Autodesk Inventor part; units mm, degrees
ref_plane "YZ Plane" through (0, 0, 0) normal (1, 0, 0) x (0, 1, 0)
ref_plane "XZ Plane" through (0, 0, 0) normal (0, 1, 0) x (-1, 0, 0)
ref_plane "XY Plane" through (0, 0, 0) normal (0, 0, 1) x (1, 0, 0)
sketch "Sketch2" plane through (0, 0, 0) normal (0, 1, 0) x (-1, 0, 0)
  line L0 (-26, 25.5) -> (26, 25.5)
  line L1 (26, 25.5) -> (26, -25.5)
  line L2 (26, -25.5) -> (-26, -25.5)
  line L3 (-26, -25.5) -> (-26, 25.5)
  line L4 (-26, 25.5) -> (26, -25.5) construction
  line L5 (26, 25.5) -> (-26, -25.5) construction
  circle A0 centre (24, 23.5) radius 1
  circle A1 centre (24, -23.5) radius 1
  circle A2 centre (-24, 23.5) radius 1
  circle A3 centre (-24, -23.5) radius 1
  line L6 (10, 6) -> (-10, 6)
  line L7 (-10, -6) -> (10, -6)
  line L8 (10, 6) -> (-10, -6) construction
  line L9 (-10, 6) -> (10, -6) construction
  line L10 (10, 6) -> (10, -6)
  line L11 (-10, 6) -> (-10, -6)
  point P0 (0, 0)
  dimension "d2" = 52
  dimension "d3" = 51
  dimension "d4" = 2
  dimension "d5" = 2
  dimension "d6" = 2
  dimension "d9" = 47
  dimension "d12" = 48
  dimension "d17" = 20
  dimension "d18" = 12
extrude "Extrusion2" add sketch "Sketch2" along normal blind 1.6
equation "\"d5\" = d4"
equation "\"d6\" = d4"
properties part number "rapoukMotherboardConnectorv0"
The listing builds one solid part. Answer for the finished solid, in the listing's coordinates (mm). A direction names the side the tool comes from. Give positions to 0.01 mm unless a question says otherwise; leave off trailing zeros. Loops run counter-clockwise (first coordinate to the right, second up) from the corner with the lowest first, then second, coordinate; pieces in that order, holes last. Notation, with made-up numbers: (42.25, 18.25) - (78.25, 18.25) arc R18 cw to (78.25, 38.25) - close; hole circle Ø5 at (45, 49.25). An arc over 180 degrees is marked (long way). Answer as CSV lines item,"result". Start each with the question number.
Item 1: A cutting plane is placed at D-D on x = 3.5. Determine the outline of the cut face in (y, z).
Item 2: This flat-tipped pin is pushed along its axis until it touches: pin 1 (1.8 mm diameter, centred on x = -24, z = 23.5, fed in from +Y). Where does it stop, or does it pass through?
Item 3: Find the intervals of material crossed by line 1 (Z direction, x = 24, y = 1.05); line 2 (Z direction, x = 6.5, y = 1), in increasing order. Write a range as from..to.
Item 4: A cutting plane is placed at B-B on z = 2. Determine the outline of the cut face in (x, y).
Item 5: A cutting plane is placed at C-C on y = 0.35. Determine the outline of the cut face in (x, z), then the cut area to 3 significant figures.
Item 6: For faces 1 (the face through (10, 1, 0)), 2 (the face through (-26, 1, 0)), determine the directions among +Z, -Z, +X, -X, +Y, -Y from which every point of the face is accessible in a straight line to the end or side of a thin tool.
Item 7: The mould has two halves that part along Z. Classify faces 3 (the face through (0, 1, -25.5)), 4 (the face through (-11, 1.6, 0)), 5 (the face through (0, 1, -6)): +Z half, -Z half, draft (parallel to the pull), parting line (faces both ways), or undercut.
Item 8: A cutting plane is placed at A-A on x = 24. Determine the outline of the cut face in (y, z).
Found:
1,outline,"(0, -25.5) - (1.6, -25.5) - (1.6, -6) - (0, -6) - close; (0, 6) - (1.6, 6) - (1.6, 25.5) - (0, 25.5) - close"
2,pin 1,"passes through"
3,line 1,"z = -25.5..-24.5, -22.5..22.5, 24.5..25.5"
3,line 2,"z = -25.5..-6, 6..25.5"
4,outline,"(-26, 0) - (-10, 0) - (-10, 1.6) - (-26, 1.6) - close; (10, 0) - (26, 0) - (26, 1.6) - (10, 1.6) - close"
5,outline,"(-26, -25.5) - (26, -25.5) - (26, 25.5) - (-26, 25.5) - close; hole circle Ø2 at (-24, -23.5); hole circle Ø2 at (-24, 23.5); hole (-10, -6) - (10, -6) - (10, 6) - (-10, 6) - close; hole circle Ø2 at (24, -23.5); hole circle Ø2 at (24, 23.5)"
5,area,"2,400 mm^2"
6,face 1,"+Y, -Y"
6,face 2,"+Z, -Z, -X, +Y, -Y"
7,face 3,"-Z half"
7,face 4,"draft"
7,face 5,"undercut"
8,outline,"(0, -25.5) - (1.6, -25.5) - (1.6, -24.5) - (0, -24.5) - close; (0, -22.5) - (1.6, -22.5) - (1.6, 22.5) - (0, 22.5) - close; (0, 24.5) - (1.6, 24.5) - (1.6, 25.5) - (0, 25.5) - close"
